from build123d import *

# Parameters (mm, degrees)
F1_DEPTH = 19
F2_SIZE  = 1.5


with BuildPart() as f1:
    # F0 (on Top) → F1 (new body)
    with BuildSketch(Plane.XY):
        Polygon((0, 20), (0, 0), (3, 0), (3, 3), (8.5, 3), (8.5, 2), (10, 2), (13, 4), (13, 5), (3, 5), (3, 10), (13, 10), (13, 11), (10, 13), (8.5, 13), (8.5, 12), (3, 12), (3, 20), align=None)
    extrude(amount=F1_DEPTH)

    # F2
    f2_edges = [f1.edges().sort_by_distance(p)[0] for p in [
        (0, 0, 9.5),
    ]]
    chamfer(f2_edges, length=F2_SIZE)


solid = f1.part
For this review, take the finished solid that the model builds, in its own axes (mm). A direction names the side the tool comes from. Round coordinates to 2 decimals unless told otherwise and drop trailing zeros. Write each loop counter-clockwise with the first axis right and the second up, starting at its lowest first coordinate (ties: lowest second). Pieces come first, ordered by that corner, then holes. Notation, with made-up numbers: (84.5, -25) - (101.5, -25) arc R19 cw to (101.5, -5) - close; hole circle Ø1 at (-24, 54.25). An arc over 180 degrees is marked (long way). Write item = value, one per line. Start each with the question number.
1. Wall thickness on L1, parallel to Y at x = 7.25, z = 4; L2, parallel to X at y = 16.5, z = 18; L3, parallel to Y at x = 9.25, z = 3.75: over which ranges is each line inside the solid? List them lowest first.
2. Consider section B-B on y = 12.75. State the section outline as (x, z) points (3 decimals).
3. Draft analysis for pull direction X (two halves, no side actions). For faces 6 (the face through (3, 7, 9)), 7 (the face through (6, 12, 9)), 8 (the face through (2, 8, 0)), 9 (the face through (8.5, 2.5, 9.4)), state which applies: released by +X, released by -X, zero draft, split by the parting line, or undercut.
4. For faces 1 (the face through (9, 2, 9)), 2 (the face through (0, 11, 9)), 3 (the face through (9, 13, 9)), 4 (the face through (8, 10, 9)), 5 (the face through (6, 3, 9)), list the 3-axis set-ups (+Z, -Z, +X, -X, +Y, -Y) from which the entire face can be reached by the end or side of a thin tool; tool diameter is ignored.
5. For pin 1 Ø1.5 at (y, z) = (1.5, 8.5) entering from +X (3 decimals); pin 2 Ø5 at (x, z) = (8.5, 5.5) entering from -Y; pin 3 Ø1 at (x, y) = (1.5, 2.5) entering from -Z; pin 4 Ø3 at (x, z) = (6.5, 11.5) entering from -Y, all flat-tipped, find the tip position at first contact; note any pin that passes through.
6. Consider section A-A on x = 9. State the section outline as (y, z) points.
7. Consider section C-C on z = 18.25. State the section outline as (x, y) points.
Evaluation:
q1.L1 = 3 to 5, 10 to 12
q1.L2 = 0 to 3
q1.L3 = 2 to 5, 10 to 13
q2.outline = (0, 0) - (3, 0) - (3, 19) - (0, 19) - close; (8.5, 0) - (10.375, 0) - (10.375, 19) - (8.5, 19) - close
q3.face_6 = released by +X
q3.face_7 = undercut
q3.face_8 = zero draft
q3.face_9 = undercut
q4.face_1 = +Z, -Z, +X, -Y
q4.face_2 = +Z, -Z, -X, +Y, -Y
q4.face_3 = +Z, -Z, +X, +Y
q4.face_4 = +Z, -Z, +X
q4.face_5 = +Z, -Z, -Y
q5.pin_1 = 10.375
q5.pin_2 = 2
q5.pin_3 = 0
q5.pin_4 = 3
q6.outline = (2, 0) - (5, 0) - (5, 19) - (2, 19) - close; (10, 0) - (13, 0) - (13, 19) - (10, 19) - close
q7.outline = (0, 1.5) - (1.5, 0) - (3, 0) - (3, 3) - (8.5, 3) - (8.5, 2) - (10, 2) - (13, 4) - (13, 5) - (3, 5) - (3, 10) - (13, 10) - (13, 11) - (10, 13) - (8.5, 13) - (8.5, 12) - (3, 12) - (3, 20) - (0, 20) - close
